Work out the finished part from the listing and answer in its coordinate system (mm). A direction names the side the tool comes from. Give positions to 0.01 mm unless a question says otherwise; leave off trailing zeros. Loops run counter-clockwise (first coordinate to the right, second up) from the corner with the lowest first, then second, coordinate; pieces in that order, holes last. Notation, with made-up numbers: (45.5, 3) - (84.5, 3) arc R22 ccw to (84.5, 22) - close; hole circle Ø7 at (73.25, -13). An arc over 180 degrees is marked (long way). One line per item, written item: value.
from build123d import *

# Parameters (mm, degrees)
F2_DEPTH  = 60
F4_DEPTH  = 5
F5_R      = 5
F6_DEPTH  = 5
F8_DEPTH  = 30.0010001
F9_R      = 20
F10_DEPTH = 60.0010001


# Not quite as in the source:
# - a pattern or mirror of a feature is missing from the dataset's text; its kind, count and spacing are read off the source's solid


with BuildPart() as f2:
    # F1 (on Front) → F2 (new body)
    with BuildSketch(Plane.XZ):
        with BuildLine():
            Line((-30, 0), (30, 0))
            ThreePointArc((30, 0), (0, 30), (-30, 0))
        make_face()
    extrude(amount=-F2_DEPTH)

    # F3 (on Top) → F4 (join)
    with BuildSketch(Plane.XY):
        with BuildLine():
            ThreePointArc((-40, 60), (-50, 50), (-40, 40))
            Line((-40, 40), (40, 40))
            ThreePointArc((40, 40), (50, 50), (40, 60))
            Line((40, 60), (-40, 60))
        make_face()
    extrude(amount=F4_DEPTH)

    # F5 (on Top) → F6 (cut, through all)
    with BuildSketch(Plane.XY):
        with Locations((-40, 50)):
            Circle(F5_R)
    f6 = extrude(amount=F6_DEPTH, mode=Mode.SUBTRACT)

    # F6_copies: F6 across plane
    add(f6.mirror(Plane(origin=(0, 0, 0), x_dir=(0, 0, 1), z_dir=(1, 0, 0))), mode=Mode.SUBTRACT)

    # F7 (on Top) → F8 (cut, through all)
    with BuildSketch(Plane.XY):
        with BuildLine():
            Line((-10, 20), (-10, 0))
            Line((-10, 0), (0, 0))
            Line((0, 0), (0, 30))
            ThreePointArc((0, 30), (-7.0710678119, 27.0710678119), (-10, 20))
        make_face()
        with BuildLine():
            Line((0, 30), (0, 0))
            Line((0, 0), (10, 0))
            Line((10, 0), (10, 20))
            ThreePointArc((10, 20), (7.0710678119, 27.0710678119), (0, 30))
        make_face()
    extrude(amount=F8_DEPTH, mode=Mode.SUBTRACT)

    # F9 (on face) → F10 (cut, through all)
    with BuildSketch(Plane.XZ):
        Circle(F9_R)
    extrude(amount=-F10_DEPTH, mode=Mode.SUBTRACT)


solid = f2.part
1. For faces 4 (the cylindrical face through (-50, 50, 2)), 5 (the flat face through (-35, 48, 5)), 6 (the flat face through (35, 48, 5)), 7 (the flat face through (10, 10, 23)), 8 (the flat face through (1, 60, 21)), determine the directions among +Z, -Z, +X, -X, +Y, -Y from which every point of the face is accessible in a straight line to the end or side of a thin tool.
Output:
face 4: +Z, -Z, -X
face 5: +Z, -X, +Y, -Y
face 6: +Z, +X, +Y, -Y
face 7: +Z, -Z, -Y
face 8: +Z, -Z, +X, -X, +Y
2. Section B-B (y = 50) is taken. Write down the section's boundary in (x, z).
Output:
outline: (-50, 0) - (-45, 0) - (-45, 5) - (-50, 5) - close; (-35, 0) - (-20, 0) arc R20 cw to (20, 0) - (35, 0) - (35, 5) - (29.58, 5) arc R30 ccw to (-29.58, 5) - (-35, 5) - close; (45, 0) - (50, 0) - (50, 5) - (45, 5) - close
3. Find the intervals of material crossed by line 1 along Y through (x, z) = (-40, 2.65); line 2 along X through (y, z) = (10.5, 27); line 3 along X through (y, z) = (56, 12.5), in increasing order.
Output:
line 1: y = 40 to 45, 55 to 60
line 2: x = -13.08 to -10, 10 to 13.08
line 3: x = -27.27 to -15.61, 15.61 to 27.27
4. Flat-ended cylindrical pins translate along their axes: pin 1 Ø9 at (x, y) = (40, 50) entering from -Z; pin 2 Ø10 at (x, y) = (9.5, 35) entering from +Z; pin 3 Ø12 at (y, z) = (41.5, 23) entering from +X; pin 4 Ø12 at (y, z) = (11.5, 20.5) entering from -X. Find the tip coordinate at first contact, or state that the pin passes through.
Output:
pin 1: passes through
pin 2: stops at z = 29.66
pin 3: stops at x = 24.72
pin 4: stops at x = -26.26
5. Section D-D (z = 26) is taken. Write down the section's boundary in (x, y).
Output:
outline: (-14.97, 0) - (-10, 0) - (-10, 20) arc R10 cw to (10, 20) - (10, 0) - (14.97, 0) - (14.97, 60) - (-14.97, 60) - close
6. Section A-A (z = 4) is taken. Write down the section's boundary in (x, y).
Output:
outline: (-40, 40) - (-29.73, 40) - (-29.73, 0) - (-19.6, 0) - (-19.6, 60) - (-40, 60) arc R10 ccw to start; (19.6, 0) - (29.73, 0) - (29.73, 40) - (40, 40) arc R10 ccw to (40, 60) - (19.6, 60) - close; hole circle Ø10 at (-40, 50); hole circle Ø10 at (40, 50)
7. The mould has two halves that part along Y. Classify faces 1 (the flat face through (-29, 37, 0)), 2 (the flat face through (20, 0, 14)), 3 (the cylindrical face through (44, 53, 2)): released by +Y, released by -Y, zero draft, split by the parting line, or undercut.
Output:
face 1: zero draft
face 2: released by -Y
face 3: undercut
8. Section C-C (y = 10.5) is taken. Write down the section's boundary in (x, z).
Output:
outline: (-30, 0) - (-20, 0) arc R20 cw to (-10, 17.32) - (-10, 28.28) arc R30 ccw to start; (10, 17.32) arc R20 cw to (20, 0) - (30, 0) arc R30 ccw to (10, 28.28) - close
